Design review of the part built by this model. Coordinates are the model's own, in mm. A direction names the side the tool comes from. Round coordinates to 2 decimals unless told otherwise and drop trailing zeros. Write each loop counter-clockwise with the first axis right and the second up, starting at its lowest first coordinate (ties: lowest second). Pieces come first, ordered by that corner, then holes. Notation, with made-up numbers: (35.5, 79.5) -> (55.5, 79.5) arc R28 cw to (55.5, 111.5) -> close; hole circle Ø2 at (16.25, 39.25). An arc over 180 degrees is marked (long way). One line per question, with ' | ' between items. Start each with the question number.
1) Mouldability with a two-part tool opening along Y and no side actions: class faces 1 (the flat face through (1, 8, -0.358)), 2 (the cylindrical face through (1.55, 0.19, 2.03)), 3 (the conical face through (-1.44, 10.87, -1.46)), 4 (the flat face through (0, -0.51, 0)) as +Y half, -Y half, draft (parallel to the pull), parting line (faces both ways), or undercut.
2) Consider section A-A (y = 8.75). Give the boundary of the cut face in (x, z).
3) Insertion check: pin 1 Ø2 at (y, z) = (8.5, -1.5) entering from -X; pin 2 Ø1 at (x, y) = (-1.5, 6.5) entering from -Z; pin 3 Ø1 at (x, y) = (-1.5, 6.5) entering from +Z; pin 4 Ø2 at (x, z) = (-1, -2) entering from +Y. Each pin has a flat end and moves straight along its axis. Give the tip position at first contact, or say it passes through.
4) Consider section B-B (y = 2.25). Give the boundary of the cut face in (x, z).
5) Consider section C-C (y = 4.5). Give the boundary of the cut face in (x, z).
6) For faces 5 (the cylindrical face through (1.421, 5.904, 1.446)), 6 (the cylindrical face through (-1.446, 5.904, 1.421)), 7 (the conical face through (-1.52, 7.07, -1.55)), 8 (the cylindrical face through (1.446, 5.904, -1.421)), 9 (the cylindrical face through (1.54, 9.97, 1.57)), list the 3-axis set-ups (+Z, -Z, +X, -X, +Y, -Y) from which the entire face can be reached by the end or side of a thin tool; tool diameter is ignored.
7) For probe 1 along Y at (x, z) = (0, -1.5); probe 2 along Y at (x, z) = (2, -2); probe 3 along Z at (x, y) = (-1, 10.5), list the stretches that pass through material, from the lowest coordinate up.
```python
from build123d import *

# Parameters (mm, degrees)
SLITCUTSKE_W       = 5.33220965
SLITCUTSKE_H       = 0.7155
SLITCUT_DEPTH      = 6.8582
SLITCUTPAT_COUNT   = 2
SLITCUTPAT_ANGLE   = 90
CLINCHCUT_START    = -1.345
CLINCHCUT_DEPTH    = 1.345
CLINCHCUTPAT_COUNT = 30
CLINCHCUTPAT_ANGLE = 348


with BuildPart() as part:
    # BodySke → Body (revolve)
    with BuildSketch(Plane.XY, mode=Mode.PRIVATE) as body_sk:
        Polygon((2.5555, 0), (2.5555, 0.3825), (2.87, 0.3825), (2.87, 1.5475), (2.69, 1.7275), (2.69, 4.18905), (2.02725, 4.8518), (2.02725, 6.92675), (2.385, 7.2845), (2.385, 8), (2, 8), (2.2, 9.79), (2.2, 10.148), (1.9, 11.58), (0, 11.58), (0, -0.51), (3.175, -0.51), (3.175, 0), align=None)
    revolve(body_sk.sketch.rotate(Axis((0, -0.51, 0), (0, 1, 0)), 90), axis=Axis((0, -0.51, 0), (0, 1, 0)))

    # SlitCutSke → SlitCut (cut)
    with BuildSketch(Plane(origin=(0, 11.58, 0), x_dir=(-1, 0, 0), z_dir=(0, 1, 0))):
        Rectangle(SLITCUTSKE_W, SLITCUTSKE_H)
    slitcut = extrude(amount=-SLITCUT_DEPTH, mode=Mode.SUBTRACT)

    # SlitCutPat: SlitCut ×2 about axis
    slitcutpat_axis = Axis((0, -0.51, 0), (0, 1, 0))
    for i in range(1, SLITCUTPAT_COUNT):
        add(slitcut.rotate(slitcutpat_axis, i * SLITCUTPAT_ANGLE / (SLITCUTPAT_COUNT - 1)), mode=Mode.SUBTRACT)

    # CliRinCutSke → ClinchCut (cut)
    with BuildSketch(Plane.XZ.offset(-0.3825).offset(CLINCHCUT_START)):
        with BuildLine():
            Line((0.29999669, 2.85427784), (0, 2.69))
            Line((0, 2.69), (-0.29999669, 2.85427784))
            ThreePointArc((-0.29999669, 2.85427784), (0, 2.87), (0.29999669, 2.85427784))
        make_face()
    clinchcut = extrude(amount=CLINCHCUT_DEPTH, mode=Mode.SUBTRACT)

    # ClinchCutPat: ClinchCut ×30 about axis
    clinchcutpat_axis = Axis((0, -0.51, 0), (0, 1, 0))
    for i in range(1, CLINCHCUTPAT_COUNT):
        add(clinchcut.rotate(clinchcutpat_axis, i * CLINCHCUTPAT_ANGLE / (CLINCHCUTPAT_COUNT - 1)), mode=Mode.SUBTRACT)


solid = part.part
```
From the geometry:
1) face 1: draft | face 2: undercut | face 3: +Y half | face 4: -Y half
2) outline: (-2.05, -0.36) arc R2.08 ccw to (-0.36, -2.05) -> (-0.36, -0.36) -> close; (-2.05, 0.36) -> (-0.36, 0.36) -> (-0.36, 2.05) arc R2.08 ccw to start; (0.36, -2.05) arc R2.08 ccw to (2.05, -0.36) -> (0.36, -0.36) -> close; (0.36, 0.36) -> (2.05, 0.36) arc R2.08 ccw to (0.36, 2.05) -> close
3) pin 1: stops at x = -2.3 | pin 2: stops at z = -1.76 | pin 3: stops at z = 1.76 | pin 4: stops at y = 11.58
4) outline: circle Ø5.38 at (0, 0)
5) outline: circle Ø4.76 at (0, 0)
6) face 5: +Z, +X | face 6: +Z, -X | face 7: -Z, -X | face 8: -Z, +X | face 9: +Z, +X, +Y
7) probe 1: y = -0.51 to 4.72 | probe 2: y = -0.51 to 0 | probe 3: z = -1.88 to -0.36, 0.36 to 1.88
